Could you check a few things on this model? Use its own coordinates, in mm. A direction names the side the tool comes from. Round coordinates to 2 decimals unless told otherwise and drop trailing zeros. Write each loop counter-clockwise with the first axis right and the second up, starting at its lowest first coordinate (ties: lowest second). Pieces come first, ordered by that corner, then holes. Notation, with made-up numbers: (63.25, 22.25) -> (81.25, 22.25) arc R23 ccw to (81.25, 38.25) -> close; hole circle Ø2 at (69, 18). An arc over 180 degrees is marked (long way). One line per question, with ' | ' between items. Start each with the question number.
1. Imagine slicing it at D-D, the plane z = -2. List the corners of the cut face in (x, y) for me, and give its area (3 significant figures).
2. Imagine slicing it at B-B, the plane z = 18. List the corners of the cut face in (x, y) for me, and give its area (3 significant figures).
3. For faces 1 (the flat face through (0, -62, -5)), 2 (the flat face through (-5, -62, 50.286)), 3 (the cylindrical face through (43.346, -12.503, 34.868)), 4 (the flat face through (24, -62, 70.286)), 5 (the flat face through (39, -62, 52)), which set-ups out of +Z, -Z, +X, -X, +Y, -Y let a thin tool reach every point of the face, with its end or its side?
4. Imagine slicing it at A-A, the plane y = -95.5. List the corners of the cut face in (x, z) for me, and give its area (3 significant figures).
5. Imagine slicing it at C-C, the plane x = 19.5. List the corners of the cut face in (y, z) for me, and give its area (3 significant figures).
6. If I drill on line 1 along Z through (x, y) = (44.5, -48); line 2 along X through (y, z) = (-8, 12.5); line 3 along Z through (x, y) = (8, -58.5), over which ranges is the centre line in solid material (lowest first)? Write a range as [from, to].
7. For pin 1 Ø11.5 at (x, y) = (20, -90.5) entering from +Z; pin 2 Ø2.5 at (x, y) = (42, -48) entering from -Z; pin 3 Ø10 at (y, z) = (-66, 44.5) entering from -X, each with a flat end and sliding along its axis, tell me the tip position at first contact or that it passes through.
8. Thinking about a two-plate mould opening in X: for faces 6 (the flat face through (47.571, -62, 50)), 7 (the flat face through (23, -62, 0)), 8 (the flat face through (0, -62, 55)), which applies, released by +X, released by -X, zero draft, split by the parting line, or undercut?
from build123d import *

# Parameters (mm, degrees)
F1_DEPTH = 125
F3_DEPTH = 25


with BuildPart() as f1:
    # F0 (on Front) → F1 (new body)
    with BuildSketch(Plane.XZ):
        Polygon((0, -10), (0, 0), (47.57143, 0), (47.57143, 70.285714), (0, 70.285714), (0, 80.285714), (-10, 80.285714), (-10, 50.285714), (0, 50.285714), (0, 60.285714), (38.999996, 60.285714), (38.999996, 10), (0, 10), (0, 20), (-10, 20), (-10, -10), align=None)
    extrude(amount=F1_DEPTH)

    # F2 (on face) → F3 (cut)
    with BuildSketch(Plane.YZ.offset(47.57143)):
        with BuildLine():
            Line((-25, 47.642857), (-100, 47.642857))
            ThreePointArc((-100, 47.642857), (-112.5, 35.142857), (-100, 22.642857))
            Line((-100, 22.642857), (-25, 22.642857))
            ThreePointArc((-25, 22.642857), (-12.5, 35.142857), (-25, 47.642857))
        make_face()
    extrude(amount=-F3_DEPTH, mode=Mode.SUBTRACT)


solid = f1.part
Geometry results:
1) outline: (-10, -125) -> (0, -125) -> (0, 0) -> (-10, 0) -> close | area: 1,250 mm2
2) outline: (-10, -125) -> (0, -125) -> (0, 0) -> (-10, 0) -> close; (39, -125) -> (47.57, -125) -> (47.57, 0) -> (39, 0) -> close | area: 2,320 mm2
3) face 1: -Z, +X, +Y, -Y | face 2: -X, +Y, -Y | face 3: +X, -X | face 4: +Z, +X, +Y, -Y | face 5: +Y, -Y
4) outline: (-10, -10) -> (0, -10) -> (0, 0) -> (47.57, 0) -> (47.57, 22.64) -> (39, 22.64) -> (39, 10) -> (0, 10) -> (0, 20) -> (-10, 20) -> close; (-10, 50.29) -> (0, 50.29) -> (0, 60.29) -> (39, 60.29) -> (39, 47.64) -> (47.57, 47.64) -> (47.57, 70.29) -> (0, 70.29) -> (0, 80.29) -> (-10, 80.29) -> close | area: 1,770 mm2
5) outline: (-125, 0) -> (0, 0) -> (0, 10) -> (-125, 10) -> close; (-125, 60.29) -> (0, 60.29) -> (0, 70.29) -> (-125, 70.29) -> close | area: 2,500 mm2
6) line 1: z = [0, 22.64], [47.64, 70.29] | line 2: x = [-10, 0], [39, 47.57] | line 3: z = [0, 10], [60.29, 70.29]
7) pin 1: stops at z = 70.29 | pin 2: stops at z = 0 | pin 3: stops at x = 39
8) face 6: released by +X | face 7: zero draft | face 8: undercut
